For this review, take the finished solid that the model builds, in its own axes (mm). A direction names the side the tool comes from. Round coordinates to 2 decimals unless told otherwise and drop trailing zeros. Order: outer loops, then holes, each group sorted by start corner. A loop starts at its lowest first (then second) coordinate and runs counter-clockwise, first axis right, second up. Notation, with made-up numbers: M 65.25,84 L 118.25,84 A13 cw 118.25,98 Z; hole C 7,42.25 d7. An arc over 180 degrees is marked long. Put each result on its own line as item: value.
from build123d import *

# Parameters (mm, degrees)
F0_W     = 500
F0_H     = 190
F1_DEPTH = 50
F2_W     = 500
F2_H     = 300
F3_DEPTH = 20
F4_W     = 500
F4_H     = 20
F5_DEPTH = 170


# Not quite as in the source:
# - the program builds the solid bodies; features that only make, move or delete a surface that nothing else refers to are left out


with BuildPart() as f1:
    # F0 (on Top) → F1 (new body)
    with BuildSketch(Plane.XY):
        with Locations((0, -95)):
            Rectangle(F0_W, F0_H)
    extrude(amount=-F1_DEPTH)

    # F2 (on Front) → F3 (join)
    with BuildSketch(Plane.XZ):
        with Locations((0, -150)):
            Rectangle(F2_W, F2_H)
    extrude(amount=F3_DEPTH)

    # F4 (on face) → F5 (join)
    with BuildSketch(Plane.XZ.offset(20)):
        with Locations((0, -240)):
            Rectangle(F4_W, F4_H)
    extrude(amount=F5_DEPTH)


solid = f1.part
(1) Add section A-A on y = -106. Give the boundary of the cut face in (x, z).
A:
outline: M -250,-250 L 250,-250 L 250,-230 L -250,-230 Z; M -250,-50 L 250,-50 L 250,0 L -250,0 Z
(2) Draft analysis for pull direction Z (two halves, no side actions). For faces 4 (the face through (-3, -20, -139)), 5 (the face through (250, -17, -95)), 6 (the face through (-3, -104, -250)), state which applies: released by +Z, released by -Z, zero draft, split by the parting line, or undercut.
A:
face 4: undercut
face 5: zero draft
face 6: released by -Z
(3) Add section C-C on z = -199.5. Give the boundary of the cut face in (x, y), then the cut area to 3 significant figures.
A:
outline: M -250,-20 L 250,-20 L 250,0 L -250,0 Z
area: 10,000 mm2
(4) Add section B-B on x = 209. Give the boundary of the cut face in (y, z).
A:
outline: M -190,-250 L -20,-250 L -20,-300 L 0,-300 L 0,0 L -190,0 L -190,-50 L -20,-50 L -20,-230 L -190,-230 Z
(5) Insertion check: pin 1 Ø12 at (y, z) = (-134, -57.5) entering from +X; pin 2 Ø3 at (x, z) = (-124.5, -115.5) entering from -Y; pin 3 Ø4 at (x, y) = (190.5, -34) entering from -Z. Each pin has a flat end and moves straight along its axis. Give the tip position at first contact, or say it passes through.
A:
pin 1: passes through
pin 2: stops at y = -20
pin 3: stops at z = -250
(6) To check wall thickness, follow L1, parallel to Z at x = 142, y = -105.5; L2, parallel to Y at x = -90.5, z = -198. State the ranges of each line that lie inside material, in increasing order.
A:
L1: z = -250 to -230, -50 to 0
L2: y = -20 to 0
(7) For faces 1 (the face through (-3, -20, -275)), 2 (the face through (-3, -104, -230)), 3 (the face through (-3, -10, -300)), list the 3-axis set-ups (+Z, -Z, +X, -X, +Y, -Y) from which the entire face can be reached by the end or side of a thin tool; tool diameter is ignored.
A:
face 1: -Z, +X, -X, -Y
face 2: +X, -X, -Y
face 3: -Z, +X, -X, +Y, -Y
